Source: CAD feature listing. Evaluate the final solid. Frame: model axes, mm. A direction names the side the tool comes from. Coordinates: 2 decimals unless noted, no trailing zeros. Loops run counter-clockwise (first coordinate to the right, second up) from the corner with the lowest first, then second, coordinate; pieces in that order, holes last.
from build123d import *

# Parameters (mm, degrees)
F2_R = 2


with BuildPart() as f1:
    # F0 (on Right) → F1 (revolve)
    with BuildSketch(Plane.YZ):
        with BuildLine():
            Line((27.72, 25), (27.72, 0))
            Line((27.72, 0), (48, 0))
            Line((48, 0), (48, 38))
            ThreePointArc((48, 38), (39.310272, 38.023274), (30.820276, 36.170745))
            ThreePointArc((30.820276, 36.170745), (25.882203, 32.529384), (24, 26.689746))
            Line((24, 26.689746), (24, 25))
            Line((24, 25), (27.72, 25))
        make_face()
    revolve(axis=Axis((0, 0, 20.223878), (0, 0, 1)))

    # F2
    f2_edges = [f1.edges().sort_by_distance(p)[0] for p in [
        (0, -48, 38),
        (0, -27.72, 0),
    ]]
    fillet(f2_edges, radius=F2_R)


solid = f1.part
Q1. Line query: line 1 along Y through (x, z) = (0, 8); line 2 along Y through (x, z) = (0, 26.25). Output: solid intervals per line, ascending.
Q2. Contact query for flat-ended pins moving along their axis: pin 1 Ø1.5 at (x, y) = (7, 27.5) entering from -Z; pin 2 Ø1.5 at (x, z) = (-19.5, 29) entering from -Y; pin 3 Ø2 at (x, z) = (23, 12) entering from +Y. Output: stop coordinate, or through.
Q3. Draft query along X for faces 3 (the cylindrical face through (-23.374, 14.902, 13.339)), 4 (the flat face through (21, 22, 0)), 5 (the cylindrical face through (46.859, -10.405, 18.338)). Return one class per face: +X half, -X half, draft (parallel to the pull), parting line (faces both ways), or undercut.
Q4. Section A-A, the plane z = 5. Return the cut outline in (x, y), plus the area to 3 significant figures.
Q5. Access query for faces 1 (the cylindrical face through (-1.055, -23.977, 25.833)), 2 (the flat face through (-23, 8, 25)). Directions: +Z, -Z, +X, -X, +Y, -Y. A direction counts if a zero-diameter tool reaches every point of the face in a straight line with its end or side. Return the directions, or none.
Derived:
1. line 1: y = -48 to -27.72, 27.72 to 48
1. line 2: y = -48 to -24, 24 to 48
2. pin 1: stops at z = 0.09
2. pin 2: stops at y = -44.19
2. pin 3: stops at y = 42.66
3. face 3: undercut
3. face 4: draft
3. face 5: parting line
4. outline: circle Ø96 at (0, 0); hole circle Ø55.44 at (0, 0)
4. area: 4,820 mm2
5. face 1: +Z, -Z
5. face 2: -Z
